Input: part model. Units: mm. Frame: model coordinates. A direction names the side the tool comes from. Coordinates: 2 decimals unless noted, no trailing zeros. Order: outer loops, then holes, each group sorted by start corner. A loop starts at its lowest first (then second) coordinate and runs counter-clockwise, first axis right, second up.
from build123d import *

# Parameters (mm, degrees)
F1_DEPTH     = 31.75
F2_W         = 377.4263709784
F2_H         = 129.2024739087
F2_R         = 9.525
F3_DEPTH     = 6.35
F4_W         = 382.6104104519
F4_H         = 158.9530184865
F5_DEPTH     = 3.175
F6_R         = 12.7
F6_R_2       = 9.525
F6_R_3       = 7.9375
F7_DEPTH     = 25.4
F8_R         = 17.4625
F9_DEPTH     = 12.7
F10_S5_R     = 17.4625
F10_T6_DEPTH = 26
F11_SIZE     = 4.76249


# Not quite as in the source:
# - a fillet or chamfer that OpenCascade refuses, or shapes differently, is made with other operations: its cross-section is extruded or revolved along the edge and cut away or added
# - a fillet or chamfer is up to 0.001 mm smaller than in the source, because OpenCascade refuses the exact size


with BuildPart() as f1:
    # F0 (on Top) → F1 (new body)
    with BuildSketch(Plane.XY):
        with BuildLine():
            Line((167.4749, 50.8), (-167.4749, 50.8))
            ThreePointArc((-167.4749, 50.8), (-176.9999, 0), (-167.4749, -50.8))
            Line((-167.4749, -50.8), (167.4749, -50.8))
            ThreePointArc((167.4749, -50.8), (176.9999, 0), (167.4749, 50.8))
        make_face()
    extrude(amount=F1_DEPTH)

    # F2 (on face) → F3 (cut)
    with BuildSketch(Plane.XY.offset(31.75)):
        with Locations((2.5683268905, -4.8314835876)):
            Rectangle(F2_W, F2_H)
        Circle(F2_R, mode=Mode.SUBTRACT)
    extrude(amount=-F3_DEPTH, mode=Mode.SUBTRACT)

    # F4 (on face) → F5 (cut)
    with BuildSketch(Plane.XY.offset(25.4)):
        with Locations((2.3195892572, -0.8801557124)):
            Rectangle(F4_W, F4_H)
        with BuildLine():
            Line((-167.4749, 50.8), (-88.1336606718, 50.8))
            Line((-88.1336606718, 50.8), (88.0661393282, 50.8))
            Line((88.0661393282, 50.8), (167.4749, 50.8))
            ThreePointArc((167.4749, 50.8), (176.9999, 0), (167.4749, -50.8))
            Line((167.4749, -50.8), (88.0661393282, -50.8))
            Line((88.0661393282, -50.8), (-88.1336606718, -50.8))
            Line((-88.1336606718, -50.8), (-167.4749, -50.8))
            ThreePointArc((-167.4749, -50.8), (-176.9999, 0), (-167.4749, 50.8))
        make_face(mode=Mode.SUBTRACT)
        with BuildLine():
            Line((167.4749, 50.8), (88.0661393282, 50.8))
            ThreePointArc((88.0661393282, 50.8), (101.6675213437, 0), (88.0661393282, -50.8))
            Line((88.0661393282, -50.8), (167.4749, -50.8))
            ThreePointArc((167.4749, -50.8), (176.9999, 0), (167.4749, 50.8))
        make_face()
        with BuildLine():
            ThreePointArc((-88.1336606718, -50.8), (-101.7350426874, 0), (-88.1336606718, 50.8))
            Line((-88.1336606718, 50.8), (-167.4749, 50.8))
            ThreePointArc((-167.4749, 50.8), (-176.9999, 0), (-167.4749, -50.8))
            Line((-167.4749, -50.8), (-88.1336606718, -50.8))
        make_face()
    extrude(amount=-F5_DEPTH, mode=Mode.SUBTRACT)

    # F6 (on face) → F7 (cut)
    with BuildSketch(Plane.XY.offset(25.4)):
        with Locations((-74.6125, 0)):
            Circle(F6_R)
        with Locations((74.6125, 0)):
            Circle(F6_R)
        with Locations((114.3, 0)):
            Circle(F6_R_2)
        with Locations((157.9499, 0)):
            Circle(F6_R_2)
        with Locations((-114.3, 0)):
            Circle(F6_R_2)
        with Locations((-157.9499, 0)):
            Circle(F6_R_2)
        with Locations((-114.3, 34.925)):
            Circle(F6_R_3)
        with Locations((-114.3, -34.925)):
            Circle(F6_R_3)
        with Locations((114.3, 34.925)):
            Circle(F6_R_3)
        with Locations((114.3, -34.925)):
            Circle(F6_R_3)
    extrude(amount=-F7_DEPTH, mode=Mode.SUBTRACT)

    # F8 (on face) → F9 (cut)
    with BuildSketch(Plane(origin=(0, 0, 0), x_dir=(1, 0, 0), z_dir=(0, 0, -1))):
        with Locations((-74.6125, 0)):
            Circle(F8_R)
        with Locations((74.6125, 0)):
            Circle(F8_R)
    extrude(amount=-F9_DEPTH, mode=Mode.SUBTRACT)

    # F10: chamfer of 4.7752 on 1 edges, made by hand


with BuildPart() as f10_tool2:
    # F10_s3 → F10_t4 (revolve)
    with BuildSketch(Plane.XZ):
        Polygon((87.3125, 17.4752), (92.0877, 12.7), (87.3125, 12.7), align=None)
    revolve(axis=Axis((74.6125, 0, 12.7), (0, 0, 1)))

    # F10_s5 → F10_t6 (intersect, symmetric)
    with BuildSketch(Plane.XY.offset(15.1)):
        with Locations((74.6125, 0)):
            Circle(F10_S5_R)
    extrude(amount=F10_T6_DEPTH, both=True, mode=Mode.INTERSECT)


with BuildPart() as f1_1:
    add(f1.part)

    # F10_t1: cut F10_tool2
    add(f10_tool2.part, mode=Mode.SUBTRACT)

    # F11 (size 4.7625 in the source; OpenCascade refuses exactly that, so slightly less here)
    f11_edges = [f1_1.edges().sort_by_distance(p)[0] for p in [
        (-87.3125, 0, 12.7),
    ]]
    chamfer(f11_edges, length=F11_SIZE)


solid = f1_1.part
Item 1: Draft query along Y for faces 3 (the face through (86.726, 3.815, 21.493)), 4 (the face through (-1, 12, 25.4)), 5 (the face through (2, 50.8, 13)). Return one class per face: pulls with the +Y half, pulls with the -Y half, needs draft (parallel to the pull), parting line crosses it, or undercut.
Response values:
face 3: undercut
face 4: needs draft
face 5: pulls with the +Y half
Item 2: Cut plane A-A on x = -114.3. Return loops of the section in (y, z) (1 decimal), then the cut area to 3 significant figures.
Response values:
outline: (-50.8, 0) - (-42.9, 0) - (-42.9, 22.2) - (-50.8, 22.2) - close; (-27, 0) - (-9.5, 0) - (-9.5, 22.2) - (-27, 22.2) - close; (9.5, 0) - (27, 0) - (27, 22.2) - (9.5, 22.2) - close; (42.9, 0) - (50.8, 0) - (50.8, 22.2) - (42.9, 22.2) - close
area: 1,130 mm2
Item 3: Ray query, probe 1 along Y at (x, z) = (-114, 17); probe 2 along X at (y, z) = (-29, 18.5); probe 3 along Z at (x, y) = (-89, 14.5). Return the intervals inside material, ascending.
Response values:
probe 1: y = -50.8 to -42.86, -26.99 to -9.52, 9.52 to 26.99, 42.86 to 50.8
probe 2: x = -173.97 to -119.58, -109.02 to 109.02, 119.58 to 173.97
probe 3: z = 0 to 25.4
Item 4: Pin query (flat end, axial travel): pin 1 Ø25 at (x, y) = (157.95, 0) entering from +Z (3 decimals); pin 2 Ø3 at (x, z) = (-93, 28.5) entering from -Y; pin 3 Ø8 at (x, y) = (-83.5, -35.5) entering from +Z; pin 4 Ø10 at (y, z) = (-27, 15) entering from +X. Return the tip coordinate at first contact, or that it passes through.
Response values:
pin 1: stops at z = 22.225
pin 2: passes through
pin 3: stops at z = 25.4
pin 4: stops at x = 175.26
Item 5: Cut plane B-B on x = 156. Return loops of the section in (y, z) (3 decimals), then the cut area to 3 significant figures.
Response values:
outline: (-50.8, 0) - (-9.323, 0) - (-9.323, 22.225) - (-50.8, 22.225) - close; (9.323, 0) - (50.8, 0) - (50.8, 22.225) - (9.323, 22.225) - close
area: 1,840 mm2
Item 6: Access query for faces 1 (the face through (-57.956, -5.245, 6.261)), 2 (the face through (-122.23, 35.27, 11.27)). Directions: +Z, -Z, +X, -X, +Y, -Y. A direction counts if a zero-diameter tool reaches every point of the face in a straight line with its end or side. Return the directions, or none.
Response values:
face 1: -Z
face 2: +Z, -Z
Item 7: Cut plane C-C on z = 3. Count the separate pieces of the cut face and the enclosed holes in it, then the cut area to 3 significant figures.
Response values:
separate pieces: 1
enclosed holes: 10
area: 31,500 mm2
